Geometry: see drawing. Coordinates: mm, zero at the bounding-box minimum. A direction names the side the tool comes from. Round coordinates to 2 decimals unless told otherwise and drop trailing zeros. Order: outer loops, then holes, each group sorted by start corner. A loop starts at its lowest first (then second) coordinate and runs counter-clockwise, first axis right, second up. Notation, with made-up numbers: (20.5, 73.25) -> (38.5, 73.25) arc R6 cw to (38.5, 84.25) -> close; hole circle Ø10 at (9.5, 18.25). An arc over 180 degrees is marked (long way). Answer as CSV lines item,"result". Start each with the question number.
(1) Section query A-A (z = 3.95). Output: boundary loops of the cut face in (x, y).
(2) Line query: line 1 along X through (y, z) = (26, 4.6); line 2 along Z through (x, y) = (3, 22). Output: solid intervals per line, ascending. Write a range as from..to.
(3) Set-up query: the marked faces 1 and 2. Return all of +Z, -Z, +X, -X, +Y, -Y with unobstructed straight access to the full face (end or side cutting, diameter ignored); none if empty.
(4) Section query B-B (z = 1.75). Output: boundary loops of the cut face in (x, y).
(5) Pull-direction query (Y, two-part tool) for the marked faces 3, 4, 5 and 6; classes: +Y half, -Y half, draft (parallel to the pull), parting line (faces both ways), or undercut.
(6) Contact query for flat-ended pins moving along their axis: P1, Ø1.6, axis at x = 6, z = 3.5, coming from the -Y side; P2, Ø6, axis at x = 21.5, y = 25.5, coming from the +Z side; P3, Ø0.6, axis at x = 6.5, z = 4, coming from the +Y side; P4, Ø12, axis at x = 5, y = 18, coming from the +Z side. Output: stop coordinate, or through.
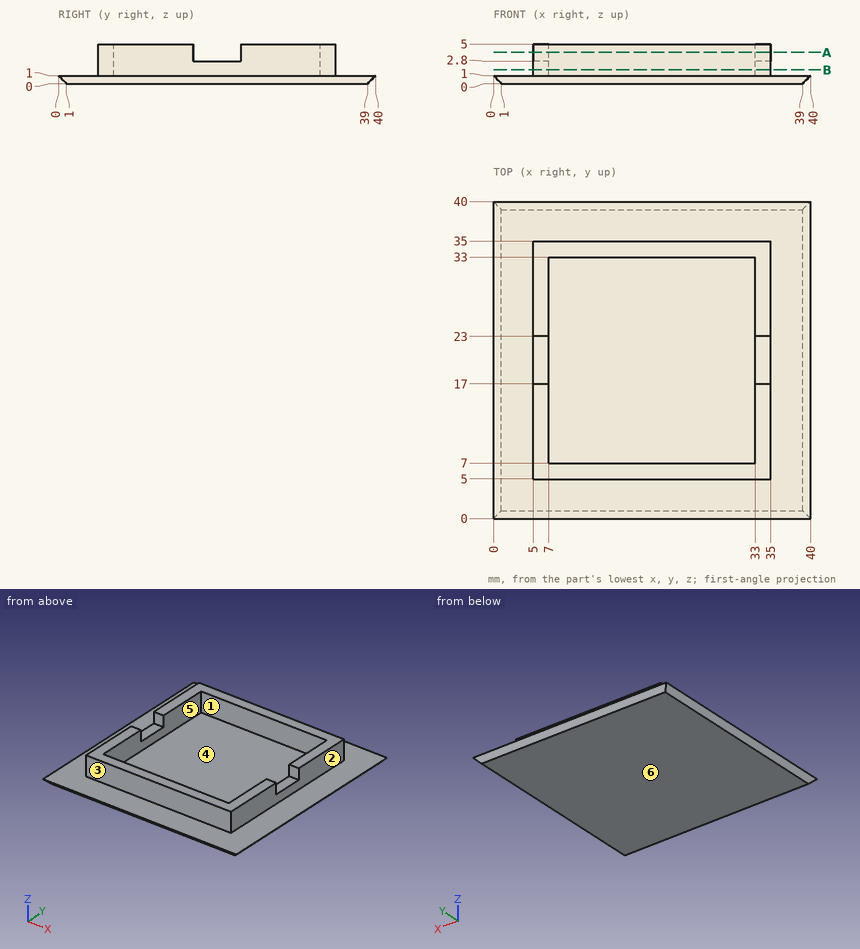
Answer block:
1,outline,"(5, 5) -> (35, 5) -> (35, 17) -> (33, 17) -> (33, 7) -> (7, 7) -> (7, 17) -> (5, 17) -> close; (5, 23) -> (7, 23) -> (7, 33) -> (33, 33) -> (33, 23) -> (35, 23) -> (35, 35) -> (5, 35) -> close"
2,line 1,"5..7, 33..35"
2,line 2,"0..1"
3,face 1,"+Z"
3,face 2,"+Z, +X, +Y, -Y"
4,outline,"(5, 5) -> (35, 5) -> (35, 35) -> (5, 35) -> close; hole (7, 7) -> (33, 7) -> (33, 33) -> (7, 33) -> close"
5,face 3,"-Y half"
5,face 4,"undercut"
5,face 5,"undercut"
5,face 6,"draft"
6,P1,"y = 5"
6,P2,"z = 1"
6,P3,"y = 35"
6,P4,"z = 5"
